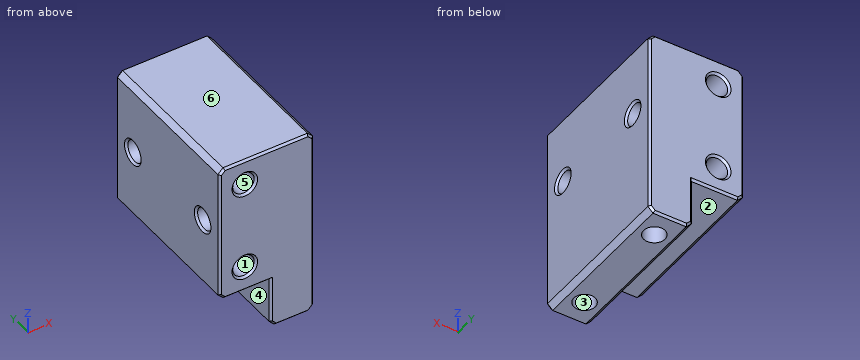
```python
from build123d import *

# Parameters (mm, degrees)
PAD022_DEPTH    = 31
SKETCH037_R     = 2.1
POCKET013_DEPTH = 31.001
SKETCH038_R     = 2.1
POCKET014_DEPTH = 16.201
SKETCH039_R     = 2.1
POCKET015_DEPTH = 18.501
CHAMFER002_SIZE = 1
CHAMFER003_SIZE = 0.4
CHAMFER004_SIZE = 0.4


with BuildPart() as sidemotorleftclone:
    # Sketch036 → Pad022 (new body)
    with BuildSketch(Plane.XZ):
        Polygon((21.5, -16.2), (21.5, 21.2), (40, 21.2), (40, -6.2), (30, -6.2), (30, -16.2), align=None)
    extrude(amount=-PAD022_DEPTH)

    # Sketch037 → Pocket013 (cut, through all)
    with BuildSketch(Plane.XZ):
        with Locations((35, 16.2)):
            Circle(SKETCH037_R)
        with Locations((35, -1.2)):
            Circle(SKETCH037_R)
    extrude(amount=-POCKET013_DEPTH, mode=Mode.SUBTRACT)

    # Sketch038 → Pocket014 (cut, through all)
    with BuildSketch(Plane.XY):
        with Locations((25.75, 26)):
            Circle(SKETCH038_R)
        with Locations((25.75, 5)):
            Circle(SKETCH038_R)
    extrude(amount=-POCKET014_DEPTH, mode=Mode.SUBTRACT)

    # Sketch039 (on Face9 of Pocket014) → Pocket015 (cut, through all)
    with BuildSketch(Plane(origin=(40, 0, 0), x_dir=(0, 0, 1), z_dir=(1, 0, 0))):
        with Locations((7.5, -5)):
            Circle(SKETCH039_R)
        with Locations((7.5, -26)):
            Circle(SKETCH039_R)
    extrude(amount=-POCKET015_DEPTH, mode=Mode.SUBTRACT)

    # Chamfer002
    chamfer002_edges = [sidemotorleftclone.edges().sort_by_distance(p)[0] for p in [
        (40, 15.5, 21.2),
        (21.5, 15.5, -16.2),
        (30, 15.5, -16.2),
        (40, 15.5, -6.2),
        (21.5, 15.5, 21.2),
    ]]
    chamfer(chamfer002_edges, length=CHAMFER002_SIZE)

    # Chamfer003
    chamfer003_edges = [sidemotorleftclone.edges().sort_by_distance(p)[0] for p in [
        (21.5, 31, 2.5),
        (22, 31, -15.7),
        (22, 31, 20.7),
        (25.75, 31, -16.2),
        (30.75, 31, 21.2),
        (29.5, 31, -15.7),
        (39.5, 31, 20.7),
        (30, 31, -10.7),
        (40, 31, 7.5),
        (34.5, 31, -6.2),
        (39.5, 31, -5.7),
        (32.9, 31, -1.2),
        (32.9, 31, 16.2),
        (21.5, 0, 2.5),
        (22, 0, -15.7),
        (22, 0, 20.7),
        (25.75, 0, -16.2),
        (30.75, 0, 21.2),
        (29.5, 0, -15.7),
        (39.5, 0, 20.7),
        (30, 0, -10.7),
        (40, 0, 7.5),
        (34.5, 0, -6.2),
        (39.5, 0, -5.7),
        (32.9, 0, -1.2),
        (32.9, 0, 16.2),
    ]]
    chamfer(chamfer003_edges, length=CHAMFER003_SIZE)

    # Chamfer004
    chamfer004_edges = [sidemotorleftclone.edges().sort_by_distance(p)[0] for p in [
        (40, 5, 5.4),
        (40, 26, 5.4),
        (21.5, 5, 5.4),
        (21.5, 26, 5.4),
    ]]
    chamfer(chamfer004_edges, length=CHAMFER004_SIZE)


with BuildPart() as part_mirroring:
    # Part__Mirroring: instance of SideMotorLeftClone
    add(sidemotorleftclone.part.mirror(Plane(origin=(0, 0, 0), x_dir=(0, -1, 0), z_dir=(1, 0, 0))))


solid = part_mirroring.part
```
Could you check a few things on this model? Use its own coordinates, in mm. Face numbers are marked on the shaded views. A direction names the side the tool comes from. Coordinates: 2 decimals unless noted, no trailing zeros. Write each loop counter-clockwise with the first axis right and the second up, starting at its lowest first coordinate (ties: lowest second). Pieces come first, ordered by that corner, then holes. Notation, with made-up numbers: (-30, 8) -> (-5, 8) arc R18 ccw to (-5, 27) -> close; hole circle Ø1 at (40.5, -18). An arc over 180 degrees is marked (long way). Write item = value, one per line. Start each with the question number.
(1) Will these pins go through, and if not, where does the flat tip stop? pin 1 (2.5 mm diameter, centred on x = -32.5, y = 8, fed in from -Z); pin 2 (2.5 mm diameter, centred on x = -35, z = 16.2, fed in from -Y); pin 3 (4.5 mm diameter, centred on y = 9.5, z = -11, fed in from -X); pin 4 (2.5 mm diameter, centred on x = -25.75, y = 5, fed in from -Z).
(2) Which directions (+Z, -Z, +X, -X, +Y, -Y) give clear straight access to the entire face, cutting with the end or side of a thin tool? Please do the marked faces 1, 2 and 3.
(3) I want a section at C-C (y = 5). Please give me the cut outline in (x, z).
(4) I want a section at B-B (x = -35). Please give me the cut outline in (y, z).
(5) I need wall thicknesses on line 1 (Z direction, x = -35, y = 17.5); line 2 (Y direction, x = -25.75, z = -3.75); line 3 (Z direction, x = -31, y = 5). Which ranges of each line are inside material? Lowest first, please. Write a range as [from, to].
(6) We'd pull the mould along Z, two halves only. Please class the marked faces 4, 5 and 6: released by +Z, released by -Z, zero draft, split by the parting line, or undercut.
(7) I want a section at A-A (z = -1.2). Please give me the cut outline in (x, y).
(8) I want a section at D-D (z = 7.5). Please give me the cut outline in (x, y), plus the area to 3 significant figures.
Result set:
q1.pin_1 = -6.2
q1.pin_2 = through
q1.pin_3 = -30
q1.pin_4 = 0
q2.face_1 = +Y, -Y
q2.face_2 = -Z, -X, +Y, -Y
q2.face_3 = -Z
q3.outline = (-40, -5.2) -> (-39, -6.2) -> (-30, -6.2) -> (-30, -15.2) -> (-29, -16.2) -> (-27.85, -16.2) -> (-27.85, 0) -> (-23.65, 0) -> (-23.65, -16.2) -> (-22.5, -16.2) -> (-21.5, -15.2) -> (-21.5, 5) -> (-21.9, 5.4) -> (-39.6, 5.4) -> (-40, 5) -> close; (-40, 10) -> (-39.6, 9.6) -> (-21.9, 9.6) -> (-21.5, 10) -> (-21.5, 20.2) -> (-22.5, 21.2) -> (-39, 21.2) -> (-40, 20.2) -> close; hole circle Ø4.2 at (-35, -1.2); hole circle Ø4.2 at (-35, 16.2)
q4.outline = (0, -5.8) -> (0.4, -6.2) -> (30.6, -6.2) -> (31, -5.8) -> (31, -3.7) -> (30.6, -3.3) -> (0.4, -3.3) -> (0, -3.7) -> close; (0, 1.3) -> (0.4, 0.9) -> (30.6, 0.9) -> (31, 1.3) -> (31, 13.7) -> (30.6, 14.1) -> (0.4, 14.1) -> (0, 13.7) -> close; (0, 18.7) -> (0.4, 18.3) -> (30.6, 18.3) -> (31, 18.7) -> (31, 20.8) -> (30.6, 21.2) -> (0.4, 21.2) -> (0, 20.8) -> close; hole circle Ø4.2 at (5, 7.5); hole circle Ø4.2 at (26, 7.5)
q5.line_1 = [-6.2, -3.3], [0.9, 14.1], [18.3, 21.2]
q5.line_2 = [0, 2.9], [7.1, 23.9], [28.1, 31]
q5.line_3 = [-6.2, 5.4], [9.6, 21.2]
q6.face_4 = zero draft
q6.face_5 = undercut
q6.face_6 = released by +Z
q7.outline = (-40, 0.4) -> (-39.6, 0) -> (-37.5, 0) -> (-37.1, 0.4) -> (-37.1, 30.6) -> (-37.5, 31) -> (-39.6, 31) -> (-40, 30.6) -> close; (-32.9, 0.4) -> (-32.5, 0) -> (-21.9, 0) -> (-21.5, 0.4) -> (-21.5, 30.6) -> (-21.9, 31) -> (-32.5, 31) -> (-32.9, 30.6) -> close; hole circle Ø4.2 at (-25.75, 5); hole circle Ø4.2 at (-25.75, 26)
q8.outline = (-40, 0.4) -> (-39.6, 0) -> (-21.9, 0) -> (-21.5, 0.4) -> (-21.5, 2.5) -> (-21.9, 2.9) -> (-39.6, 2.9) -> (-40, 2.5) -> close; (-40, 7.5) -> (-39.6, 7.1) -> (-21.9, 7.1) -> (-21.5, 7.5) -> (-21.5, 23.5) -> (-21.9, 23.9) -> (-39.6, 23.9) -> (-40, 23.5) -> close; (-40, 28.5) -> (-39.6, 28.1) -> (-21.9, 28.1) -> (-21.5, 28.5) -> (-21.5, 30.6) -> (-21.9, 31) -> (-39.6, 31) -> (-40, 30.6) -> close
q8.area = 417 mm2
